```python
from build123d import *

# Parameters (mm, degrees)
F0_W     = 112
F0_H     = 50.5
F1_DEPTH = 20
F2_R     = 5
F4_D     = 4.1
F6_DEPTH = 20
F7_W     = 58.122847
F7_H     = 6
F8_DEPTH = 1


with BuildPart() as f1:
    # F0 (on Top) → F1 (new body)
    with BuildSketch(Plane.XY):
        Polygon((80, 3), (-80, 3), (-80, -3), (-62, -3), (-62, -59.5), (62, -59.5), (62, -3), (80, -3), align=None)
        with Locations((0, -28.25)):
            Rectangle(F0_W, F0_H, mode=Mode.SUBTRACT)
    extrude(amount=F1_DEPTH)

    # F2
    f2_edges = [f1.edges().sort_by_distance(p)[0] for p in [
        (62, -59.5, 10),
        (-62, -59.5, 10),
        (-80, -3, 10),
        (80, -3, 10),
    ]]
    fillet(f2_edges, radius=F2_R)

    # F4 (through all)
    with Locations(Plane(origin=(0, 3, 0), x_dir=(-1, 0, 0), z_dir=(0, 1, 0))):
        with Locations((-72, 10), (72, 10)):
            Hole(F4_D / 2)

    # F5 (on face) → F6 (cut, through all)
    with BuildSketch(Plane.XY.offset(20)):
        with BuildLine():
            Line((0, -55.17533), (9.8, -55.17533))
            Line((9.8, -55.17533), (9.8, -57.87533))
            Line((9.8, -57.87533), (0, -57.87533))
            Line((0, -57.87533), (0, -59.5))
            Line((0, -59.5), (57, -59.5))
            ThreePointArc((57, -59.5), (60.535534, -58.035534), (62, -54.5))
            Line((62, -54.5), (62, -3))
            Line((62, -3), (75, -3))
            ThreePointArc((75, -3), (78.535534, -1.535534), (80, 2))
            Line((80, 2), (80, 3))
            Line((80, 3), (0, 3))
            Line((0, 3), (0, 1.5))
            Line((0, 1.5), (-10, 1.5))
            Line((-10, 1.5), (-10, -1.5))
            Line((-10, -1.5), (0, -1.5))
            Line((0, -1.5), (0, -3))
            Line((0, -3), (56, -3))
            Line((56, -3), (56, -53.5))
            Line((56, -53.5), (0, -53.5))
            Line((0, -53.5), (0, -55.17533))
        make_face()
    extrude(amount=-F6_DEPTH, mode=Mode.SUBTRACT)

    # F7 (on face) → F8 (join)
    with BuildSketch(Plane(origin=(0, 3, 0), x_dir=(-1, 0, 0), z_dir=(0, 1, 0))):
        with Locations((37.804018, 10)):
            Rectangle(F7_W, F7_H)
    extrude(amount=F8_DEPTH)


solid = f1.part
```
Verification items for the finished model (mm, model axes). A direction names the side the tool comes from. Give positions to 0.01 mm unless a question says otherwise; leave off trailing zeros. Order: outer loops, then holes, each group sorted by start corner. A loop starts at its lowest first (then second) coordinate and runs counter-clockwise, first axis right, second up. Notation, with made-up numbers: (-26, 24) -> (15, 24) arc R18 ccw to (15, 58) -> close; hole circle Ø3 at (14.25, -0.75). An arc over 180 degrees is marked (long way). One line per item, written item: value.
(1) Gauge pin test, flat ends, axial feed: pin 1 (1.6 mm diameter, centred on y = -2.5, z = 11.5, fed in from +X); pin 2 (0.5 mm diameter, centred on x = -27.5, y = 3.5, fed in from +Z); pin 3 (0.5 mm diameter, centred on y = 3.5, z = 11.5, fed in from +X). Record the tip position at first contact, or that the pin passes through.
Final values:
pin 1: x = 0
pin 2: z = 13
pin 3: x = -8.74
(2) Scan lines: line 1 along Y through (x, z) = (-5, 11.25); line 2 along Z through (x, y) = (-72, -0.7); line 3 along Y through (x, z) = (-22, 18.5). Record each from-to range of solid material in increasing order. Write a range as [from, to].
Final values:
line 1: [-59.5, -53.5], [-3, -1.5], [1.5, 3]
line 2: [0, 7.95], [12.05, 20]
line 3: [-59.5, -53.5], [-3, 3]
(3) Sectioned sample at D-D on y = -40. Record the cut outline in (x, z), then the cut area to 3 significant figures.
Final values:
outline: (-62, 0) -> (-56, 0) -> (-56, 20) -> (-62, 20) -> close
area: 120 mm^2
(4) Sectioned sample at C-C on z = 18.5. Record the cut outline in (x, y), then the cut area to 3 significant figures.
Final values:
outline: (-80, 2) arc R5 ccw to (-75, -3) -> (-62, -3) -> (-62, -54.5) arc R5 ccw to (-57, -59.5) -> (0, -59.5) -> (0, -57.88) -> (9.8, -57.88) -> (9.8, -55.18) -> (0, -55.18) -> (0, -53.5) -> (-56, -53.5) -> (-56, -3) -> (0, -3) -> (0, -1.5) -> (-10, -1.5) -> (-10, 1.5) -> (0, 1.5) -> (0, 3) -> (-80, 3) -> close
area: 1,140 mm^2
(5) Tool access check on faces 1 (the face through (5, -57.875, 10)), 2 (the face through (-69, -3, 10)), 3 (the face through (-59, -28, 0)), 4 (the face through (-5, -1.5, 10)), 5 (the face through (-37, 4, 10)). Record the directions out of +Z, -Z, +X, -X, +Y, -Y that give a thin tool (end or side, any length) a straight path to the whole face; none if there is none.
Final values:
face 1: +Z, -Z, +X, -Y
face 2: +Z, -Z, -X, -Y
face 3: -Z, +X, -X, +Y, -Y
face 4: +Z, -Z, +X
face 5: +Z, -Z, +X, -X, +Y
(6) Draft check along Y on faces 6 (the face through (-62, -28, 10)), 7 (the face through (5, -55.175, 10)), 8 (the face through (-28, -53.5, 10)). Enter one of: pulls with the +Y half, pulls with the -Y half, needs draft (parallel to the pull), parting line crosses it, or undercut.
Final values:
face 6: needs draft
face 7: pulls with the +Y half
face 8: undercut
(7) Sectioned sample at B-B on x = -72. Record the cut outline in (y, z), then the cut area to 3 significant figures.
Final values:
outline: (-3, 0) -> (3, 0) -> (3, 7.95) -> (-3, 7.95) -> close; (-3, 12.05) -> (3, 12.05) -> (3, 20) -> (-3, 20) -> close
area: 95.4 mm^2
(8) Sectioned sample at A-A on z = 10. Record the cut outline in (x, y), then the cut area to 3 significant figures.
Final values:
outline: (-80, 2) arc R5 ccw to (-75, -3) -> (-74.05, -3) -> (-74.05, 3) -> (-80, 3) -> close; (-69.95, -3) -> (-62, -3) -> (-62, -54.5) arc R5 ccw to (-57, -59.5) -> (0, -59.5) -> (0, -57.88) -> (9.8, -57.88) -> (9.8, -55.18) -> (0, -55.18) -> (0, -53.5) -> (-56, -53.5) -> (-56, -3) -> (0, -3) -> (0, -1.5) -> (-10, -1.5) -> (-10, 1.5) -> (0, 1.5) -> (0, 3) -> (-8.74, 3) -> (-8.74, 4) -> (-66.87, 4) -> (-66.87, 3) -> (-69.95, 3) -> close
area: 1,170 mm^2
